Here's how the part is built. I have some questions about the finished solid (model axes, mm). Face numbers are marked on the shaded views. A direction names the side the tool comes from. Give positions to 0.01 mm unless a question says otherwise; leave off trailing zeros. Write each loop counter-clockwise with the first axis right and the second up, starting at its lowest first coordinate (ties: lowest second). Pieces come first, ordered by that corner, then holes. Notation, with made-up numbers: (88.5, 42) -> (146.5, 42) arc R16 ccw to (146.5, 49) -> close; hole circle Ø4 at (-6, 29.5). An arc over 180 degrees is marked (long way). Use CSV: the item, a comma, the result in double quotes. Start each with the question number.
(1) If we mould it in two halves opening along X, with no side actions, what happens to the marked faces 1, 2 and 3? For each: pulls with the +X half, pulls with the -X half, needs draft (parallel to the pull), parting line crosses it, or undercut.
(2) Suppose I cut it at A-A on x = 5. List the corners of the cut face in (y, z) for me, plus the area to 3 significant figures.
(3) Which directions (+Z, -Z, +X, -X, +Y, -Y) give clear straight access to the entire face, cutting with the end or side of a thin tool? Please do the marked faces 4 and 5.
(4) Suppose I cut it at D-D on y = 4.5. List the corners of the cut face in (x, z) for me.
(5) For pin 1 Ø2.5 at (x, z) = (5, -26) entering from +Y; pin 2 Ø5 at (x, y) = (5, -4.5) entering from -Z; pin 3 Ø5 at (x, z) = (5, -14) entering from -Y, each with a flat end and sliding along its axis, tell me the tip position at first contact or that it passes through.
(6) Suppose I cut it at C-C on y = -7.75. List the corners of the cut face in (x, z) for me, plus the area to 3 significant figures.
(7) I need wall thicknesses on L1, parallel to X at y = -3.5, z = -4.25; L2, parallel to Z at x = 5.75, y = 3; L3, parallel to X at y = 5.5, z = -26. Which ranges of each line are inside material? Lowest first, please. Write a range as [from, to].
(8) Suppose I cut it at B-B on z = -4.25. List the corners of the cut face in (x, y) for me, plus the area to 3 significant figures.
from build123d import *

# Parameters (mm, degrees)
SKETCH1_W           = 10
SKETCH1_H           = 30
SKETCH1_R           = 2.1
BOSS_EXTRUDE1_DEPTH = 7
SKETCH2_W           = 10
SKETCH2_H           = 8
BOSS_EXTRUDE2_DEPTH = 12
SKETCH3_R           = 1.7
CUT_EXTRUDE1_DEPTH  = 37.891733491


with BuildPart() as part:
    # Sketch1 → Boss-Extrude1 (new body)
    with BuildSketch(Plane(origin=(0, 0, 0), x_dir=(1, 0, 0), z_dir=(0, 1, 0))):
        with Locations((5, 15)):
            Rectangle(SKETCH1_W, SKETCH1_H)
        with Locations(Location((5, 26, 0), (0, 0, 270))):
            Circle(SKETCH1_R, mode=Mode.SUBTRACT)
    extrude(amount=BOSS_EXTRUDE1_DEPTH)

    # Sketch2 → Boss-Extrude2 (add)
    with BuildSketch(Plane(origin=(0, 0, 0), x_dir=(-1, 0, 0), z_dir=(0, -1, 0))):
        with Locations((-5, 4)):
            Rectangle(SKETCH2_W, SKETCH2_H)
    extrude(amount=BOSS_EXTRUDE2_DEPTH)

    # Sketch3 → Cut-Extrude1 (cut, through all)
    with BuildSketch(Plane(origin=(0, 7, 0), x_dir=(1, 0, 0), z_dir=(0, 1, 0))):
        with Locations(Location((5, 4.25, 0), (0, 0, 270))):
            Circle(SKETCH3_R)
    extrude(amount=-CUT_EXTRUDE1_DEPTH, mode=Mode.SUBTRACT)


solid = part.part
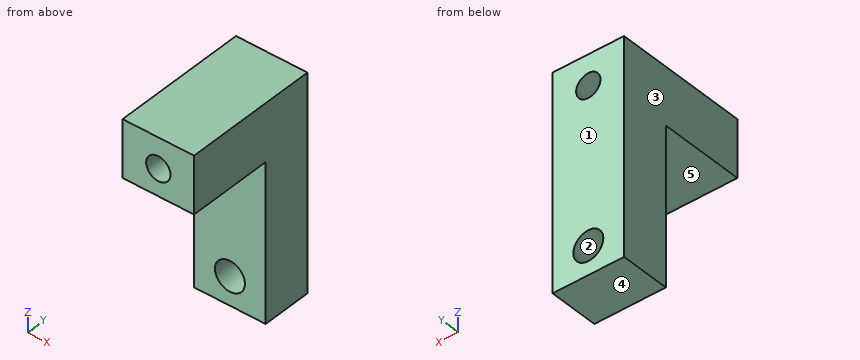
Geometry says:
1,face 1,"needs draft"
1,face 2,"undercut"
1,face 3,"pulls with the -X half"
2,outline,"(-12, -8) -> (0, -8) -> (0, -23.9) -> (7, -23.9) -> (7, -5.95) -> (-12, -5.95) -> close; (-12, -2.55) -> (7, -2.55) -> (7, 0) -> (-12, 0) -> close; (0, -30) -> (7, -30) -> (7, -28.1) -> (0, -28.1) -> close"
2,area,"212 mm²"
3,face 4,"-Z, +X, -X, +Y, -Y"
3,face 5,"-Z, +X, -X, -Y"
4,outline,"(0, -30) -> (10, -30) -> (10, 0) -> (0, 0) -> close; hole circle Ø4.2 at (5, -26); hole circle Ø3.4 at (5, -4.25)"
5,pin 1,"through"
5,pin 2,"z = -8"
5,pin 3,"y = 0"
6,outline,"(0, -8) -> (10, -8) -> (10, 0) -> (0, 0) -> close; hole circle Ø3.4 at (5, -4.25)"
6,area,"70.9 mm²"
7,L1,"[0, 3.3], [6.7, 10]"
7,L2,"[-30, -27.96], [-24.04, -5.78], [-2.72, 0]"
7,L3,"[0, 2.9], [7.1, 10]"
8,outline,"(0, -12) -> (3.3, -12) -> (3.3, 7) -> (0, 7) -> close; (6.7, -12) -> (10, -12) -> (10, 7) -> (6.7, 7) -> close"
8,area,"125 mm²"
